Build history of the part. All positions in model axes, mm. Round coordinates to 2 decimals unless told otherwise and drop trailing zeros. Order: outer loops, then holes, each group sorted by start corner. A loop starts at its lowest first (then second) coordinate and runs counter-clockwise, first axis right, second up. Notation, with made-up numbers: (64.5, -16.5) -> (85.5, -16.5) arc R9 cw to (85.5, -5.5) -> close; hole circle Ø5 at (68, 53). An arc over 180 degrees is marked (long way). Use a Markdown table: item, result. Add a question column.
Item 1: Slice it at C-C, the plane z = -48.5. Give the cut face in (x, y).
Item 2: Slice it at D-D, the plane y = 13. Give the cut face in (x, z) (3 decimals), plus the area to 3 significant figures.
Item 3: Slice it at A-A, the plane y = 19.05. Give the cut face in (x, z) (3 decimals), plus the area to 3 significant figures.
Item 4: Slice it at B-B, the plane x = -1. Give the cut face in (y, z), plus the area to 3 significant figures.
Item 5: Probe L1, parallel to X at y = 23.5, z = -26; L2, parallel to X at y = 18.25, z = -25; L3, parallel to Z at x = -3.5, y = 23.75. List the from-to ranges inside material, lowest first.
Item 6: Pin check, flat tip, straight feed: pin 1 (3 mm diameter, centred on x = -4.44, z = -26.11, fed in from -Y). Stop position of the tip, or through.
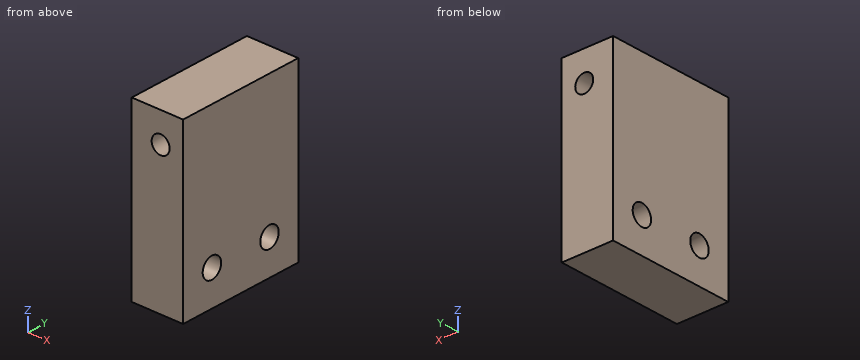
from build123d import *

# Parameters (mm, degrees)
SKETCH1_W           = 10.16
SKETCH1_H           = 25.4
SKETCH1_R           = 1.776811913
BOSS_EXTRUDE1_DEPTH = 25.4
SKETCH2_W           = 10.16
SKETCH2_H           = 25.4
BOSS_EXTRUDE2_DEPTH = 5.08
SKETCH4_W           = 10.16
SKETCH4_H           = 25.4
BOSS_EXTRUDE3_DEPTH = 3.81
SKETCH3_R           = 2.032
CUT_EXTRUDE1_DEPTH  = 62.036581459


with BuildPart() as part:
    # Sketch1 → Boss-Extrude1 (new body)
    with BuildSketch(Plane(origin=(0, 0, 0), x_dir=(1, 0, 0), z_dir=(0, 1, 0))):
        with Locations((-5.08, 32.972612439)):
            Rectangle(SKETCH1_W, SKETCH1_H)
        with Locations(Location((-4.445, 26.114612439, 0), (0, 0, 270))):
            Circle(SKETCH1_R, mode=Mode.SUBTRACT)
    extrude(amount=BOSS_EXTRUDE1_DEPTH)

    # Sketch2 → Boss-Extrude2 (add)
    with BuildSketch(Plane(origin=(0, 0, -45.672612439), x_dir=(-1, 0, 0), z_dir=(0, 0, -1))):
        with Locations((5.08, 12.7)):
            Rectangle(SKETCH2_W, SKETCH2_H)
    extrude(amount=BOSS_EXTRUDE2_DEPTH)

    # Sketch4 → Boss-Extrude3 (add)
    with BuildSketch(Plane(origin=(0, 0, -50.752612439), x_dir=(-1, 0, 0), z_dir=(0, 0, -1))):
        with Locations((5.08, 12.7)):
            Rectangle(SKETCH4_W, SKETCH4_H)
    extrude(amount=BOSS_EXTRUDE3_DEPTH)

    # Sketch3 → Cut-Extrude1 (cut, through all)
    with BuildSketch(Plane.ZY.offset(10.16)):
        with Locations((-47.704612439, 19.05)):
            Circle(SKETCH3_R)
        with Locations((-47.704612439, 6.35)):
            Circle(SKETCH3_R)
    extrude(amount=-CUT_EXTRUDE1_DEPTH, mode=Mode.SUBTRACT)


solid = part.part
Check sheet entries:
| question | item | result |
|---|---|---|
| 1 | outline | (-10.16, 0) -> (0, 0) -> (0, 4.48) -> (-10.16, 4.48) -> close; (-10.16, 8.22) -> (0, 8.22) -> (0, 17.18) -> (-10.16, 17.18) -> close; (-10.16, 20.92) -> (0, 20.92) -> (0, 25.4) -> (-10.16, 25.4) -> close |
| 2 | outline | (-10.16, -54.563) -> (0, -54.563) -> (0, -20.273) -> (-10.16, -20.273) -> close; hole circle Ø3.554 at (-4.445, -26.115) |
| 2 | area | 338 mm2 |
| 3 | outline | (-10.16, -54.563) -> (0, -54.563) -> (0, -49.737) -> (-10.16, -49.737) -> close; (-10.16, -45.673) -> (0, -45.673) -> (0, -20.273) -> (-10.16, -20.273) -> close; hole circle Ø3.554 at (-4.445, -26.115) |
| 3 | area | 297 mm2 |
| 4 | outline | (0, -54.56) -> (25.4, -54.56) -> (25.4, -20.27) -> (0, -20.27) -> close; hole circle Ø4.06 at (6.35, -47.7); hole circle Ø4.06 at (19.05, -47.7) |
| 4 | area | 845 mm2 |
| 5 | L1 | -10.16 to -6.22, -2.67 to 0 |
| 5 | L2 | -10.16 to -5.83, -3.06 to 0 |
| 5 | L3 | -54.56 to -27.62, -24.61 to -20.27 |
| 6 | pin 1 | through |
